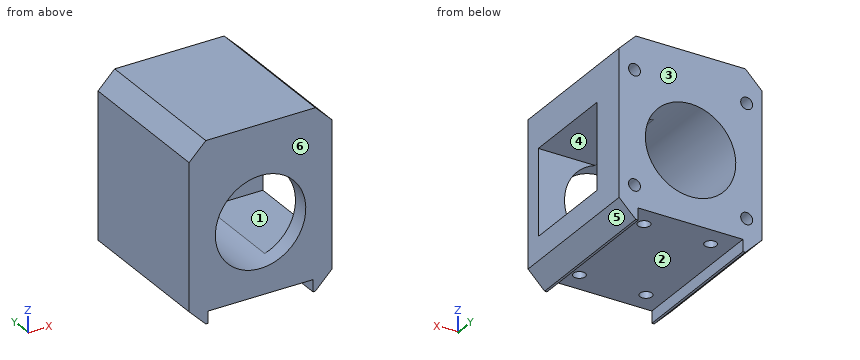
from build123d import *

# Parameters (mm, degrees)
SKETCH1_W               = 60
SKETCH1_H               = 75
BOSS_EXTRUDE1_DEPTH     = 62
SKETCH2_R               = 19
SKETCH2_W               = 44
SKETCH2_H               = 5
CUT_EXTRUDE1_DEPTH      = 62
CUT_EXTRUDE2_REACH      = 96.076
CUT_EXTRUDE2_END_RADIUS = 19
SKETCH3_W               = 36
SKETCH3_H               = 40
CHAMFER1_SIZE           = 7
SKETCH4_R               = 2.5
CUT_EXTRUDE3_DEPTH      = 10
SKETCH5_R               = 2.5
CUT_EXTRUDE4_DEPTH      = 20


with BuildPart() as part:
    # Sketch1 → Boss-Extrude1 (new body)
    with BuildSketch(Plane(origin=(0, 0, 0), x_dir=(1, 0, 0), z_dir=(0, 1, 0))):
        Rectangle(SKETCH1_W, SKETCH1_H)
    extrude(amount=BOSS_EXTRUDE1_DEPTH)

    # Sketch2 → Cut-Extrude1 (cut)
    with BuildSketch(Plane(origin=(0, 62, 0), x_dir=(1, 0, 0), z_dir=(0, 1, 0))):
        with Locations(Location((0, 2.5, 0), (0, 0, 270))):
            Circle(SKETCH2_R)
        with Locations((0, 35)):
            Rectangle(SKETCH2_W, SKETCH2_H)
    extrude(amount=-CUT_EXTRUDE1_DEPTH, mode=Mode.SUBTRACT)

    # Cut-Extrude2: up to this cylinder (the profile starts outside it)
    cut_extrude2_end = Plane(origin=(0, 27, -2.5), z_dir=(0, 1, 0)) * Cylinder(CUT_EXTRUDE2_END_RADIUS, 231.152, mode=Mode.PRIVATE)
    # Sketch3 → Cut-Extrude2 (cut, up to the surface)
    with BuildSketch(Plane(origin=(30, 0, 0), x_dir=(0, 0, -1), z_dir=(1, 0, 0)), mode=Mode.PRIVATE) as cut_extrude2_sk1:
        with Locations((2.5, 27)):
            Rectangle(SKETCH3_W, SKETCH3_H)
    cut_extrude2_tool1 = extrude(cut_extrude2_sk1.sketch, amount=-CUT_EXTRUDE2_REACH, mode=Mode.PRIVATE) - cut_extrude2_end
    add(cut_extrude2_tool1.solids().sort_by_distance((30, 27, -2.5))[0], mode=Mode.SUBTRACT)

    # Chamfer1
    chamfer1_edges = [part.edges().sort_by_distance(p)[0] for p in [
        (30, 31, 37.5),
        (-30, 31, 37.5),
        (-30, 31, -37.5),
        (30, 31, -37.5),
    ]]
    chamfer(chamfer1_edges, length=CHAMFER1_SIZE)

    # Sketch4 → Cut-Extrude3 (cut)
    with BuildSketch(Plane(origin=(0, 0, -32.5), x_dir=(-1, 0, 0), z_dir=(0, 0, -1))):
        with Locations((-14, 53)):
            Circle(SKETCH4_R)
        with Locations((14, 53)):
            Circle(SKETCH4_R)
        with Locations((-14, 9)):
            Circle(SKETCH4_R)
        with Locations((14, 9)):
            Circle(SKETCH4_R)
    extrude(amount=-CUT_EXTRUDE3_DEPTH, mode=Mode.SUBTRACT)

    # Sketch5 → Cut-Extrude4 (cut)
    with BuildSketch(Plane(origin=(0, 62, 0), x_dir=(1, 0, 0), z_dir=(0, 1, 0))):
        with Locations(Location((-23.55, 23.55, 0), (0, 0, 270))):
            Circle(SKETCH5_R)
        with Locations(Location((23.55, 23.55, 0), (0, 0, 270))):
            Circle(SKETCH5_R)
        with Locations(Location((23.55, -23.55, 0), (0, 0, 270))):
            Circle(SKETCH5_R)
        with Locations(Location((-23.55, -23.55, 0), (0, 0, 270))):
            Circle(SKETCH5_R)
    extrude(amount=-CUT_EXTRUDE4_DEPTH, mode=Mode.SUBTRACT)


solid = part.part
Design review of the part built by this model. Coordinates are the model's own, in mm. Face numbers are marked on the shaded views. A direction names the side the tool comes from. Give positions to 0.01 mm unless a question says otherwise; leave off trailing zeros. Loops run counter-clockwise (first coordinate to the right, second up) from the corner with the lowest first, then second, coordinate; pieces in that order, holes last. Notation, with made-up numbers: (53.5, -39) -> (89.5, -39) arc R23 ccw to (89.5, -6) -> close; hole circle Ø4 at (6.25, 67.25). An arc over 180 degrees is marked (long way). One line per question, with ' | ' between items. Start each with the question number.
(1) For the marked faces 1, 2 and 3, list the 3-axis set-ups (+Z, -Z, +X, -X, +Y, -Y) from which the entire face can be reached by the end or side of a thin tool; tool diameter is ignored.
(2) Insertion check: P1, Ø1.5, axis at x = -14.5, y = 8, coming from the -Z side; P2, Ø1.5, axis at x = -22.5, z = -23, coming from the +Y side; P3, Ø10, axis at y = 25.5, z = 5.5, coming from the +X side. Each pin has a flat end and moves straight along its axis. Give the tip position at first contact, or say it passes through.
(3) We need section C-C (x = 0). State the section outline as (y, z) points.
(4) Draft analysis for pull direction Y (two halves, no side actions). For the marked faces 4, 5 and 6, state which applies: +Y half, -Y half, draft (parallel to the pull), parting line (faces both ways), or undercut.
(5) We need section D-D (z = 23.55). State the section outline as (x, y) points.
(6) For line 1 (X direction, y = 58.25, z = 23.55); line 2 (Y direction, x = -14, z = -27); line 3 (Y direction, x = 21.5, z = 1.5), list the stretches that pass through material, from the lowest coordinate up.
(7) We need section A-A (y = 53). State the section outline as (x, z) points.
(8) We need section B-B (z = -23.55). State the section outline as (x, y) points.
The answers:
1) face 1: +X | face 2: -Z, +Y, -Y | face 3: +Z, -Z, +X, -X, +Y
2) P1: stops at z = -22.5 | P2: stops at y = 42 | P3: stops at x = -13.86
3) outline: (0, -32.5) -> (62, -32.5) -> (62, -21.5) -> (0, -21.5) -> close; (0, 16.5) -> (62, 16.5) -> (62, 37.5) -> (0, 37.5) -> close
4) face 4: undercut | face 5: draft | face 6: -Y half
5) outline: (-30, 0) -> (30, 0) -> (30, 62) -> (26.05, 62) -> (26.05, 42) -> (21.05, 42) -> (21.05, 62) -> (-21.05, 62) -> (-21.05, 42) -> (-26.05, 42) -> (-26.05, 62) -> (-30, 62) -> close
6) line 1: x = -30 to -26.05, -21.05 to 21.05, 26.05 to 30 | line 2: y = 0 to 6.5, 11.5 to 50.5, 55.5 to 62 | line 3: y = 0 to 7, 47 to 62
7) outline: (-30, -30.5) -> (-23, -37.5) -> (-22, -37.5) -> (-22, -32.5) -> (-16.5, -32.5) -> (-16.5, -22.5) -> (-11.5, -22.5) -> (-11.5, -32.5) -> (11.5, -32.5) -> (11.5, -22.5) -> (16.5, -22.5) -> (16.5, -32.5) -> (22, -32.5) -> (22, -37.5) -> (23, -37.5) -> (30, -30.5) -> (30, 30.5) -> (23, 37.5) -> (-23, 37.5) -> (-30, 30.5) -> close; hole circle Ø5 at (-23.55, -23.55); hole circle Ø5 at (-23.55, 23.55); hole circle Ø38 at (0, -2.5); hole circle Ø5 at (23.55, -23.55); hole circle Ø5 at (23.55, 23.55)
8) outline: (-30, 0) -> (30, 0) -> (30, 62) -> (26.05, 62) -> (26.05, 42) -> (21.05, 42) -> (21.05, 62) -> (-21.05, 62) -> (-21.05, 42) -> (-26.05, 42) -> (-26.05, 62) -> (-30, 62) -> close; hole circle Ø5 at (-14, 9); hole circle Ø5 at (-14, 53); hole circle Ø5 at (14, 9); hole circle Ø5 at (14, 53)
